The listing builds one solid part. Answer for the finished solid, in the listing's coordinates (mm). A direction names the side the tool comes from. Round coordinates to 2 decimals unless told otherwise and drop trailing zeros. Loops run counter-clockwise (first coordinate to the right, second up) from the corner with the lowest first, then second, coordinate; pieces in that order, holes last. Notation, with made-up numbers: (-18, 48.5) - (-2, 48.5) arc R16 ccw to (-2, 71.5) - close; hole circle Ø3 at (-37.5, 32.5). An arc over 180 degrees is marked (long way). One line per item, written item: value.
```python
from build123d import *

# Parameters (mm, degrees)
SKETCH_1_R      = 2
EXTRUDE_1_DEPTH = 3
EXTRUDE_START   = -3
EXTRUDE_2_DEPTH = 3


with BuildPart() as part:
    # 草图1 → 凸台-拉伸1 (new body)
    with BuildSketch(Plane(origin=(0, 0, 0), x_dir=(1, 0, 0), z_dir=(0, 1, 0))):
        with BuildLine():
            ThreePointArc((-0.804164412, 11.973024664), (-8.485281374, -8.485281374), (11.973024664, -0.804164412))
            add(Edge.make_bspline(
                [(13, 0), (12.923284361, -0.311828909), (12.495573917, -0.491752354), (12.082770065, -0.660295948), (11.973024664, -0.804164412)],
                knots=[0, 0, 0, 0, 0.61500276, 1, 1, 1, 1], degree=3))
            add(Edge.make_bspline(
                [(13, 0), (12.923284361, 0.311828909), (12.495573917, 0.491752354), (12.082770065, 0.660295948), (11.973024664, 0.804164412)],
                knots=[0, 0, 0, 0, 0.61500276, 1, 1, 1, 1], degree=3))
            ThreePointArc((11.973024664, 0.804164412), (11.954336377, 1.045868913), (11.930769201, 1.287146566))
            add(Edge.make_bspline(
                [(12.802500789, 2.25742631), (12.781099155, 1.937013252), (12.391129972, 1.685552109), (12.013864826, 1.447886434), (11.930769201, 1.287146566)],
                knots=[0, 0, 0, 0, 0.61500276, 1, 1, 1, 1], degree=3))
            add(Edge.make_bspline(
                [(12.802500789, 2.25742631), (12.672802111, 2.551196306), (12.220346171, 2.65411517), (11.78454645, 2.748415572), (11.651485831, 2.871041262)],
                knots=[0, 0, 0, 0, 0.61500276, 1, 1, 1, 1], degree=3))
            ThreePointArc((11.651485831, 2.871041262), (11.591109915, 3.105828541), (11.526003353, 3.339348247))
            add(Edge.make_bspline(
                [(12.21600407, 4.446261863), (12.250566718, 4.127000245), (11.910187813, 3.811641924), (11.579924383, 3.51207552), (11.526003353, 3.339348247)],
                knots=[0, 0, 0, 0, 0.61500276, 1, 1, 1, 1], degree=3))
            add(Edge.make_bspline(
                [(12.21600407, 4.446261863), (12.037263182, 4.713046894), (11.573809391, 4.73583404), (11.128255354, 4.753025979), (10.975922497, 4.850682976)],
                knots=[0, 0, 0, 0, 0.61500276, 1, 1, 1, 1], degree=3))
            ThreePointArc((10.975922497, 4.850682976), (10.875693444, 5.071419141), (10.771025725, 5.290085522))
            add(Edge.make_bspline(
                [(11.258330249, 6.5), (11.347807011, 6.191590424), (11.067360624, 5.821916927), (10.794133798, 5.469551968), (10.771025725, 5.290085522)],
                knots=[0, 0, 0, 0, 0.61500276, 1, 1, 1, 1], degree=3))
            add(Edge.make_bspline(
                [(11.258330249, 6.5), (11.035978102, 6.731693937), (10.57560827, 6.673656989), (10.13383785, 6.613218097), (9.966861313, 6.682939142)],
                knots=[0, 0, 0, 0, 0.61500276, 1, 1, 1, 1], degree=3))
            ThreePointArc((9.966861313, 6.682939142), (9.829824531, 6.882917236), (9.688775931, 7.080086225))
            add(Edge.make_bspline(
                [(9.958577761, 8.356238926), (10.10024993, 8.068052261), (9.888257283, 7.655295931), (9.68036892, 7.260838847), (9.688775931, 7.080086225)],
                knots=[0, 0, 0, 0, 0.61500276, 1, 1, 1, 1], degree=3))
            add(Edge.make_bspline(
                [(9.958577761, 8.356238926), (9.699370412, 8.545801866), (9.256072642, 8.408704248), (8.831508812, 8.27247093), (8.654962091, 8.312137584)],
                knots=[0, 0, 0, 0, 0.61500276, 1, 1, 1, 1], degree=3))
            ThreePointArc((8.654962091, 8.312137584), (8.485281374, 8.485281374), (8.312137584, 8.654962091))
            add(Edge.make_bspline(
                [(8.356238926, 9.958577761), (8.545801866, 9.699370412), (8.408704248, 9.256072642), (8.27247093, 8.831508812), (8.312137584, 8.654962091)],
                knots=[0, 0, 0, 0, 0.61500276, 1, 1, 1, 1], degree=3))
            add(Edge.make_bspline(
                [(8.356238926, 9.958577761), (8.068052261, 10.10024993), (7.655295931, 9.888257283), (7.260838847, 9.68036892), (7.080086225, 9.688775931)],
                knots=[0, 0, 0, 0, 0.61500276, 1, 1, 1, 1], degree=3))
            ThreePointArc((7.080086225, 9.688775931), (6.882917236, 9.829824531), (6.682939142, 9.966861313))
            add(Edge.make_bspline(
                [(6.5, 11.258330249), (6.731693937, 11.035978102), (6.673656989, 10.57560827), (6.613218097, 10.13383785), (6.682939142, 9.966861313)],
                knots=[0, 0, 0, 0, 0.61500276, 1, 1, 1, 1], degree=3))
            add(Edge.make_bspline(
                [(6.5, 11.258330249), (6.191590424, 11.347807011), (5.821916927, 11.067360624), (5.469551968, 10.794133798), (5.290085522, 10.771025725)],
                knots=[0, 0, 0, 0, 0.61500276, 1, 1, 1, 1], degree=3))
            ThreePointArc((5.290085522, 10.771025725), (5.071419141, 10.875693444), (4.850682976, 10.975922497))
            add(Edge.make_bspline(
                [(4.446261863, 12.21600407), (4.713046894, 12.037263182), (4.73583404, 11.573809391), (4.753025979, 11.128255354), (4.850682976, 10.975922497)],
                knots=[0, 0, 0, 0, 0.61500276, 1, 1, 1, 1], degree=3))
            add(Edge.make_bspline(
                [(4.446261863, 12.21600407), (4.127000245, 12.250566718), (3.811641924, 11.910187813), (3.51207552, 11.579924383), (3.339348247, 11.526003353)],
                knots=[0, 0, 0, 0, 0.61500276, 1, 1, 1, 1], degree=3))
            ThreePointArc((3.339348247, 11.526003353), (3.105828541, 11.591109915), (2.871041262, 11.651485831))
            add(Edge.make_bspline(
                [(2.25742631, 12.802500789), (2.551196306, 12.672802111), (2.65411517, 12.220346171), (2.748415572, 11.78454645), (2.871041262, 11.651485831)],
                knots=[0, 0, 0, 0, 0.61500276, 1, 1, 1, 1], degree=3))
            add(Edge.make_bspline(
                [(2.25742631, 12.802500789), (1.937013252, 12.781099155), (1.685552109, 12.391129972), (1.447886434, 12.013864826), (1.287146566, 11.930769201)],
                knots=[0, 0, 0, 0, 0.61500276, 1, 1, 1, 1], degree=3))
            ThreePointArc((1.287146566, 11.930769201), (1.045868913, 11.954336377), (0.804164412, 11.973024664))
            add(Edge.make_bspline(
                [(0, 13), (0.311828909, 12.923284361), (0.491752354, 12.495573917), (0.660295948, 12.082770065), (0.804164412, 11.973024664)],
                knots=[0, 0, 0, 0, 0.61500276, 1, 1, 1, 1], degree=3))
            add(Edge.make_bspline(
                [(0, 13), (-0.311828909, 12.923284361), (-0.491752354, 12.495573917), (-0.660295948, 12.082770065), (-0.804164412, 11.973024664)],
                knots=[0, 0, 0, 0, 0.61500276, 1, 1, 1, 1], degree=3))
        make_face()
        with Locations(Location((0, 0, 0), (0, 0, 270))):
            Circle(SKETCH_1_R, mode=Mode.SUBTRACT)
    extrude(amount=EXTRUDE_1_DEPTH)

    # 草图2 → 凸台-拉伸2 (add)
    with BuildSketch(Plane(origin=(0, 3, 0), x_dir=(1, 0, 0), z_dir=(0, 1, 0)).offset(EXTRUDE_START)):
        with BuildLine():
            ThreePointArc((4, -11.313708499), (2.029223745, -11.827182716), (0, -12))
            Line((0, -12), (0, -37.5))
            ThreePointArc((0, -37.5), (2.236067977, -38.027864045), (4, -39.5))
            Line((4, -39.5), (4, -11.313708499))
        make_face()
        with BuildLine():
            Line((0, -37.5), (0, -12))
            ThreePointArc((0, -12), (-2.029223745, -11.827182716), (-4, -11.313708499))
            Line((-4, -11.313708499), (-4, -39.5))
            ThreePointArc((-4, -39.5), (-2.236067977, -38.027864045), (0, -37.5))
        make_face()
        with BuildLine():
            ThreePointArc((4, -39.5), (2.236067977, -38.027864045), (0, -37.5))
            Line((0, -37.5), (0, -38.5))
            ThreePointArc((0, -38.5), (1.414213562, -38.758342613), (2.645751311, -39.5))
            Line((2.645751311, -39.5), (4, -39.5))
        make_face()
        with BuildLine():
            Line((0, -38.5), (0, -37.5))
            ThreePointArc((0, -37.5), (-2.236067977, -38.027864045), (-4, -39.5))
            Line((-4, -39.5), (-2.645751311, -39.5))
            ThreePointArc((-2.645751311, -39.5), (-1.414213562, -38.758342613), (0, -38.5))
        make_face()
        with BuildLine():
            ThreePointArc((5, -42.5), (4.74341649, -40.91886117), (4, -39.5))
            Line((4, -39.5), (2.645751311, -39.5))
            ThreePointArc((2.645751311, -39.5), (3.645751311, -40.854248689), (4, -42.5))
            ThreePointArc((4, -42.5), (2.828427125, -45.328427125), (0, -46.5))
            Line((0, -46.5), (0, -47.5))
            ThreePointArc((0, -47.5), (3.535533906, -46.035533906), (5, -42.5))
        make_face()
        with BuildLine():
            Line((-2.645751311, -39.5), (-4, -39.5))
            ThreePointArc((-4, -39.5), (-4.472135955, -44.736067977), (0, -47.5))
            Line((0, -47.5), (0, -46.5))
            ThreePointArc((0, -46.5), (-3.741657387, -43.914213562), (-2.645751311, -39.5))
        make_face()
    extrude(amount=EXTRUDE_2_DEPTH)


solid = part.part
```
1) Consider L1, parallel to Z at x = 1.5, y = 2.6; L2, parallel to X at y = 1.4, z = 0; L3, parallel to Z at x = -1.25, y = 0.5. Determine where each line is inside the solid, lowest interval first.
Final values:
L1: -12.11 to -1.32, 1.32 to 38.79, 46.21 to 47.27
L2: -12 to -2, 2 to 13
L3: -11.93 to -1.56, 1.56 to 38.7, 46.3 to 47.34
2) Each of these flat-tipped pins is pushed along its axis until it touches: pin 1 Ø1.5 at (y, z) = (1, 31) entering from +X; pin 2 Ø1 at (x, z) = (-1, 40.5) entering from -Y. Where does it stop, or does it pass through?
Final values:
pin 1: x = 4
pin 2: through
3) For faces 3 (the cylindrical face through (-11.855, 1.479, -1.859)), 4 (the flat face through (4, 1, 26)), determine the directions among +Z, -Z, +X, -X, +Y, -Y from which every point of the face is accessible in a straight line to the end or side of a thin tool.
Final values:
face 3: -X, +Y, -Y
face 4: +X, +Y, -Y
4) A cutting plane is placed at C-C on x = -6. Give the vertices of the cut face in (y, z), and give its area (3 significant figures).
Final values:
outline: (0, -10.39) - (3, -10.39) - (3, 10.39) - (0, 10.39) - close
area: 62.4 mm2
5) For a pull along Z with two mould halves and no side action, classify faces 1 (the flat face through (0, 3, 10)), 2 (the flat face through (-4, 1, 25)) as released by +Z, released by -Z, zero draft, split by the parting line, or undercut.
Final values:
face 1: zero draft
face 2: undercut
6) A cutting plane is placed at A-A on y = 1.3. Give the number of separate pieces and of enclosed holes in the cut face, and give its area (3 significant figures).
Final values:
separate pieces: 1
enclosed holes: 2
area: 688 mm2
7) A cutting plane is placed at B-B on z = 28. Give the vertices of the cut face in (x, y), and give its area (3 significant figures).
Final values:
outline: (-4, 0) - (4, 0) - (4, 3) - (-4, 3) - close
area: 24.0 mm2
